Geometry: final body of the model. Coordinates: model frame, mm. A direction names the side the tool comes from. Give positions to 0.01 mm unless a question says otherwise; leave off trailing zeros. Order: outer loops, then holes, each group sorted by start corner. A loop starts at its lowest first (then second) coordinate and runs counter-clockwise, first axis right, second up. Notation, with made-up numbers: (82.5, -11.5) - (91.5, -11.5) arc R20 cw to (91.5, 25.5) - close; hole circle Ø4 at (60, 42). An arc over 180 degrees is marked (long way). Put each result on its own line as item: value. Start each with the question number.
1. First-contact query: P1, Ø15, axis at x = 1.5, y = 20.5, coming from the -Z side; P2, Ø3.5, axis at y = 26, z = -4.5, coming from the +X side. Flat tips, straight axial feed; report the tip coordinate or a pass-through.
2. Mould query, pull axis Y, two halves, no side actions, for faces 1 (the flat face through (-4, 0, 0)), 2 (the cylindrical face through (-21.99, 2.8, -5.12)), 3 (the flat face through (-4, 15, 0.5)). Classes: pulls with the +Y half, pulls with the -Y half, needs draft (parallel to the pull), parting line crosses it, or undercut.
3. Section D-D on y = 7.5. Return the cut outline in (x, z).
4. Section B-B on z = -4.5. Return the cut outline in (x, y).
5. Section C-C on x = 5.5. Return the cut outline in (y, z).
6. Set-up query: faces 4 (the cylindrical face through (12.93, 15.21, -0.1)), 5 (the flat face through (-21.5, 15, -5)). Return all of +Z, -Z, +X, -X, +Y, -Y with unobstructed straight access to the full face (end or side cutting, diameter ignored); none if empty.
7. Ray query, line 1 along X through (y, z) = (17.25, -4.5); line 2 along Z through (x, y) = (9, 17.75); line 3 along X through (y, z) = (20.5, -1.25). Return the intervals inside material, ascending. Write a range as from..to.
8. Section A-A on y = 26. Return the cut outline in (x, z), plus the area to 3 significant figures.
from build123d import *

# Parameters (mm, degrees)
BOSS_EXTRUDE1_DEPTH = 30
FILLET2_R           = 2
SKETCH3_R           = 1.5
CUT_EXTRUDE4_DEPTH  = 9
SKETCH4_R           = 1.35
CUT_EXTRUDE3_DEPTH  = 37
FILLET3_R           = 1


with BuildPart() as part:
    # Sketch1 → Boss-Extrude1 (new body)
    with BuildSketch(Plane(origin=(0, 0, 0), x_dir=(1, 0, 0), z_dir=(0, 1, 0))):
        Polygon((-21.5, 0.5), (12.5, 0.5), (12.5, 7.5), (13.5, 7.5), (13.5, 0.5), (13.5, -0.5), (-22.5, -0.5), (-22.5, 0.5), (-22.5, 7.5), (-21.5, 7.5), align=None)
    extrude(amount=BOSS_EXTRUDE1_DEPTH)

    # Fillet2
    fillet2_edges = [part.edges().sort_by_distance(p)[0] for p in [
        (13.5, 15, 0.5),
        (-22.5, 15, 0.5),
        (-21.5, 15, -0.5),
        (12.5, 15, -0.5),
    ]]
    fillet(fillet2_edges, radius=FILLET2_R)

    # Sketch3 → Cut-Extrude4 (cut, through all)
    with BuildSketch(Plane.XY.offset(0.5)):
        with Locations((-14.5, 22.5)):
            Circle(SKETCH3_R)
        with Locations((5.5, 22.5)):
            Circle(SKETCH3_R)
        with Locations((-14.5, 7.5)):
            Circle(SKETCH3_R)
        with Locations((5.5, 7.5)):
            Circle(SKETCH3_R)
    extrude(amount=-CUT_EXTRUDE4_DEPTH, mode=Mode.SUBTRACT)

    # Sketch4 → Cut-Extrude3 (cut, through all)
    with BuildSketch(Plane(origin=(13.5, 0, 0), x_dir=(0, 0, -1), z_dir=(1, 0, 0))):
        with Locations((4.5, 26)):
            Circle(SKETCH4_R)
        with Locations((4.5, 4)):
            Circle(SKETCH4_R)
    extrude(amount=-CUT_EXTRUDE3_DEPTH, mode=Mode.SUBTRACT)

    # Fillet3
    fillet3_edges = [part.edges().sort_by_distance(p)[0] for p in [
        (13, 30, -7.5),
        (-22, 0, -7.5),
        (13, 0, -7.5),
        (-22, 30, -7.5),
    ]]
    fillet(fillet3_edges, radius=FILLET3_R)


solid = part.part
Resolved:
1. P1: z = -0.5
1. P2: x = 13.5
2. face 1: pulls with the -Y half
2. face 2: undercut
2. face 3: needs draft
3. outline: (-22.5, -7.5) - (-21.5, -7.5) - (-21.5, -2.5) arc R2 cw to (-19.5, -0.5) - (-16, -0.5) - (-16, 0.5) - (-20.5, 0.5) arc R2 ccw to (-22.5, -1.5) - close; (-13, -0.5) - (4, -0.5) - (4, 0.5) - (-13, 0.5) - close; (7, -0.5) - (10.5, -0.5) arc R2 cw to (12.5, -2.5) - (12.5, -7.5) - (13.5, -7.5) - (13.5, -1.5) arc R2 ccw to (11.5, 0.5) - (7, 0.5) - close
4. outline: (-22.5, 0) - (-21.5, 0) - (-21.5, 2.65) - (-22.5, 2.65) - close; (-22.5, 5.35) - (-21.5, 5.35) - (-21.5, 24.65) - (-22.5, 24.65) - close; (-22.5, 27.35) - (-21.5, 27.35) - (-21.5, 30) - (-22.5, 30) - close; (12.5, 0) - (13.5, 0) - (13.5, 2.65) - (12.5, 2.65) - close; (12.5, 5.35) - (13.5, 5.35) - (13.5, 24.65) - (12.5, 24.65) - close; (12.5, 27.35) - (13.5, 27.35) - (13.5, 30) - (12.5, 30) - close
5. outline: (0, -0.5) - (6, -0.5) - (6, 0.5) - (0, 0.5) - close; (9, -0.5) - (21, -0.5) - (21, 0.5) - (9, 0.5) - close; (24, -0.5) - (30, -0.5) - (30, 0.5) - (24, 0.5) - close
6. face 4: +Z, +X, +Y, -Y
6. face 5: -Z, +Y, -Y
7. line 1: -22.5..-21.5, 12.5..13.5
7. line 2: -0.5..0.5
7. line 3: -22.48..-21.06, 12.06..13.48
8. outline: (-22.5, -7.5) - (-21.5, -7.5) - (-21.5, -5.85) - (-22.5, -5.85) - close; (-22.5, -3.15) - (-21.5, -3.15) - (-21.5, -2.5) arc R2 cw to (-19.5, -0.5) - (10.5, -0.5) arc R2 cw to (12.5, -2.5) - (12.5, -3.15) - (13.5, -3.15) - (13.5, -1.5) arc R2 ccw to (11.5, 0.5) - (-20.5, 0.5) arc R2 ccw to (-22.5, -1.5) - close; (12.5, -7.5) - (13.5, -7.5) - (13.5, -5.85) - (12.5, -5.85) - close
8. area: 44.6 mm^2
